from build123d import *

# Parameters (mm, degrees)
F0_R     = 3.05
F1_DEPTH = 12


with BuildPart() as f1:
    # F0 (on Right) → F1 (new body)
    with BuildSketch(Plane.YZ):
        with BuildLine():
            Line((-161.27, 0), (-1.27, 0))
            ThreePointArc((-1.27, 0), (-0.371974, 0.371974), (0, 1.27))
            Line((0, 1.27), (0, 248.73))
            ThreePointArc((0, 248.73), (-0.371974, 249.628026), (-1.27, 250))
            Line((-1.27, 250), (-161.27, 250))
            ThreePointArc((-161.27, 250), (-162.168026, 249.628026), (-162.54, 248.73))
            Line((-162.54, 248.73), (-162.54, 105))
            ThreePointArc((-162.54, 105), (-122.53496, 65.624999), (-161.27, 25))
            Line((-161.27, 25), (-161.27, 0))
        make_face()
        with Locations((-6, 6)):
            Circle(F0_R, mode=Mode.SUBTRACT)
        with Locations((-6, 110.267787)):
            Circle(F0_R, mode=Mode.SUBTRACT)
        with Locations((-156.54, 244)):
            Circle(F0_R, mode=Mode.SUBTRACT)
        with Locations((-6, 244)):
            Circle(F0_R, mode=Mode.SUBTRACT)
    extrude(amount=F1_DEPTH)


solid = f1.part
The listing builds one solid part. Answer for the finished solid, in the listing's coordinates (mm). A direction names the side the tool comes from. Give positions to 0.01 mm unless a question says otherwise; leave off trailing zeros. Order: outer loops, then holes, each group sorted by start corner. A loop starts at its lowest first (then second) coordinate and runs counter-clockwise, first axis right, second up. Notation, with made-up numbers: (78, -21) - (107, -21) arc R16 ccw to (107, 3) - close; hole circle Ø5 at (44.5, 76). An arc over 180 degrees is marked (long way). One line per item, written item: value. Start each with the question number.
1) Find the intervals of material crossed by L1, parallel to Y at x = 4.25, z = 244; L2, parallel to Z at x = 7.75, y = -6; L3, parallel to Z at x = 3.5, y = -149.5, in increasing order.
2) The mould has two halves that part along Z. Classify faces 3 (the face through (5.916, -6.661, 3.023)), 4 (the face through (12, -82, 127)), 5 (the face through (6, -80, 250)): released by +Z, released by -Z, zero draft, split by the parting line, or undercut.
3) A cutting plane is placed at D-D on y = -156.54. Give the vertices of the cut face in (x, z).
4) Given pin 1 Ø3.5 at (x, z) = (4, 16.5) entering from -Y, flat-ended and moving along its own axis, determine where the tip first touches the part or whether it passes through.
5) A cutting plane is placed at B-B on z = 6. Give the vertices of the cut face in (x, y), then the cut area to 3 significant figures.
6) A cutting plane is placed at A-A on y = -6. Give the vertices of the cut face in (x, z).
7) A cutting plane is placed at C-C on z = 244. Give the vertices of the cut face in (x, y), then the cut area to 3 significant figures.
8) A tool of negligible diameter and unlimited length cuts with its end or side. For faces 1 (the face through (5.916, -4.593, 241.294)), 2 (the face through (6, -161.27, 13)), from which of +Z, -Z, +X, -X, +Y, -Y can it reach the whole face along a straight path? Write none if from no direction.
Answer sheet:
1. L1: y = -162.54 to -159.59, -153.49 to -9.05, -2.95 to 0
1. L2: z = 0 to 2.95, 9.05 to 107.22, 113.32 to 240.95, 247.05 to 250
1. L3: z = 0 to 27.16, 102.82 to 250
2. face 3: undercut
2. face 4: zero draft
2. face 5: released by +Z
3. outline: (0, 0) - (12, 0) - (12, 25.43) - (0, 25.43) - close; (0, 104.55) - (12, 104.55) - (12, 240.95) - (0, 240.95) - close; (0, 247.05) - (12, 247.05) - (12, 250) - (0, 250) - close
4. pin 1: stops at y = -161.27
5. outline: (0, -161.27) - (12, -161.27) - (12, -9.05) - (0, -9.05) - close; (0, -2.95) - (12, -2.95) - (12, 0) - (0, 0) - close
5. area: 1,860 mm2
6. outline: (0, 0) - (12, 0) - (12, 2.95) - (0, 2.95) - close; (0, 9.05) - (12, 9.05) - (12, 107.22) - (0, 107.22) - close; (0, 113.32) - (12, 113.32) - (12, 240.95) - (0, 240.95) - close; (0, 247.05) - (12, 247.05) - (12, 250) - (0, 250) - close
7. outline: (0, -162.54) - (12, -162.54) - (12, -159.59) - (0, -159.59) - close; (0, -153.49) - (12, -153.49) - (12, -9.05) - (0, -9.05) - close; (0, -2.95) - (12, -2.95) - (12, 0) - (0, 0) - close
7. area: 1,800 mm2
8. face 1: +X, -X
8. face 2: -Z, +X, -X, -Y
